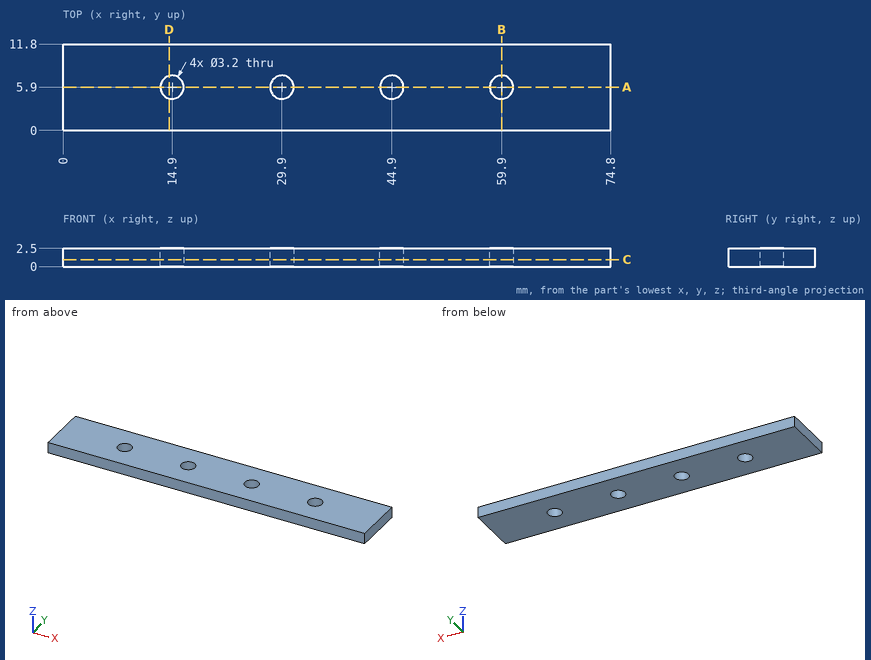
Check sheet for the drawn part. Datum: minimum x, y, z corner. Units: mm. Coordinates: 2 decimals unless noted, no trailing zeros. Loops run counter-clockwise (first coordinate to the right, second up) from the corner with the lowest first, then second, coordinate; pieces in that order, holes last. Notation, with made-up numbers: (76, 80) -> (103, 80) arc R29 cw to (103, 119) -> close; hole circle Ø8 at (71, -27.75). An arc over 180 degrees is marked (long way). Answer in a Markdown table with one row per item.
1) Scan lines: line 1 along Y through (x, z) = (29.9, 1.6); line 2 along X through (y, z) = (7, 2.25); line 3 along X through (y, z) = (4.5, 1.75). Record each from-to range of solid material in increasing order. Write a range as from..to.
The answers:
| item | result |
|---|---|
| line 1 | y = 0..4.3, 7.5..11.8 |
| line 2 | x = 0..13.74, 16.06..28.74, 31.06..43.74, 46.06..58.74, 61.06..74.8 |
| line 3 | x = 0..14.13, 15.67..29.13, 30.67..44.13, 45.67..59.13, 60.67..74.8 |
2) Depth check by flat-ended pin: P1, Ø1.9, axis at x = 59.9, y = 5.9, coming from the +Z side. Enter the tip coordinate at first touch or a pass-through.
The answers:
| item | result |
|---|---|
| P1 | passes through |
3) Section check C-C (z = 0.95). Record the cut outline in (x, y), and give its area (3 significant figures).
The answers:
| item | result |
|---|---|
| outline | (0, 0) -> (74.8, 0) -> (74.8, 11.8) -> (0, 11.8) -> close; hole circle Ø3.2 at (14.9, 5.9); hole circle Ø3.2 at (29.9, 5.9); hole circle Ø3.2 at (44.9, 5.9); hole circle Ø3.2 at (59.9, 5.9) |
| area | 850 mm2 |
4) Section check A-A (y = 5.9). Record the cut outline in (x, z), and give its area (3 significant figures).
The answers:
| item | result |
|---|---|
| outline | (0, 0) -> (13.3, 0) -> (13.3, 2.5) -> (0, 2.5) -> close; (16.5, 0) -> (28.3, 0) -> (28.3, 2.5) -> (16.5, 2.5) -> close; (31.5, 0) -> (43.3, 0) -> (43.3, 2.5) -> (31.5, 2.5) -> close; (46.5, 0) -> (58.3, 0) -> (58.3, 2.5) -> (46.5, 2.5) -> close; (61.5, 0) -> (74.8, 0) -> (74.8, 2.5) -> (61.5, 2.5) -> close |
| area | 155 mm2 |
5) Section check D-D (x = 14.5). Record the cut outline in (y, z), and give its area (3 significant figures).
The answers:
| item | result |
|---|---|
| outline | (0, 0) -> (4.35, 0) -> (4.35, 2.5) -> (0, 2.5) -> close; (7.45, 0) -> (11.8, 0) -> (11.8, 2.5) -> (7.45, 2.5) -> close |
| area | 21.8 mm2 |
6) Section check B-B (x = 59.9). Record the cut outline in (y, z), and give its area (3 significant figures).
The answers:
| item | result |
|---|---|
| outline | (0, 0) -> (4.3, 0) -> (4.3, 2.5) -> (0, 2.5) -> close; (7.5, 0) -> (11.8, 0) -> (11.8, 2.5) -> (7.5, 2.5) -> close |
| area | 21.5 mm2 |
